Verification items for the finished model (mm, model axes). Give positions to 0.01 mm unless a question says otherwise; leave off trailing zeros. Write each loop counter-clockwise with the first axis right and the second up, starting at its lowest first coordinate (ties: lowest second). Pieces come first, ordered by that corner, then holes. Notation, with made-up numbers: (74, 81.25) - (118, 81.25) arc R20 ccw to (118, 97.25) - close; hole circle Ø6 at (-35.5, -16). An arc over 180 degrees is marked (long way). Put each result on its own line as item: value.
from build123d import *

# Parameters (mm, degrees)
CROQUIS1_W              = 10
CROQUIS1_H              = 40
SALIENTE_EXTRUIR1_DEPTH = 30.26
CROQUIS2_R              = 4
CORTAR_EXTRUIR1_DEPTH   = 30.26
CROQUIS5_R              = 4
CORTAR_EXTRUIR2_DEPTH   = 15.13


with BuildPart() as part:
    # Croquis1 → Saliente-Extruir1 (new body)
    with BuildSketch(Plane(origin=(0, 0, 0), x_dir=(1, 0, 0), z_dir=(0, 1, 0))):
        Rectangle(CROQUIS1_W, CROQUIS1_H)
    extrude(amount=SALIENTE_EXTRUIR1_DEPTH)

    # Croquis2 → Cortar-Extruir1 (cut)
    with BuildSketch(Plane(origin=(0, 0, 0), x_dir=(1, 0, 0), z_dir=(0, 1, 0))):
        with Locations(Location((0, -10, 0), (0, 0, 90))):
            Circle(CROQUIS2_R)
        with Locations(Location((0, 10, 0), (0, 0, 90))):
            Circle(CROQUIS2_R)
    extrude(amount=CORTAR_EXTRUIR1_DEPTH, mode=Mode.SUBTRACT)

    # Croquis5 → Cortar-Extruir2 (cut, symmetric)
    with BuildSketch(Plane(origin=(0, 0, 0), x_dir=(0, 0, -1), z_dir=(1, 0, 0))):
        with Locations((0, 15.13)):
            Circle(CROQUIS5_R)
    extrude(amount=CORTAR_EXTRUIR2_DEPTH, both=True, mode=Mode.SUBTRACT)


solid = part.part
Q1. Go/stop test with a flat-tipped pin: pin 1 Ø7 at (y, z) = (15.13, 0) entering from -X. Record where the tip stops, or that it passes through.
Answers follow:
pin 1: passes through
Q2. Section check C-C, the plane z = 0. Record the cut outline in (x, y), plus the area to 3 significant figures.
Answers follow:
outline: (-5, 0) - (5, 0) - (5, 11.13) - (-5, 11.13) - close; (-5, 19.13) - (5, 19.13) - (5, 30.26) - (-5, 30.26) - close
area: 223 mm2
Q3. Release check for a two-part mould opening along Z. For faces 1 (the face through (0.1, 19.1, 0.5)), 2 (the face through (0, 0, 0)), 3 (the face through (0, 15, 20)) record: released by +Z, released by -Z, zero draft, split by the parting line, or undercut.
Answers follow:
face 1: undercut
face 2: zero draft
face 3: released by +Z
Q4. Scan lines: line 1 along Z through (x, y) = (-0.25, 24); line 2 along X through (y, z) = (9.5, -10); line 3 along Z through (x, y) = (1, 29). Record each from-to range of solid material in increasing order.
Answers follow:
line 1: z = -20 to -13.99, -6.01 to 6.01, 13.99 to 20
line 2: x = -5 to -4, 4 to 5
line 3: z = -20 to -13.87, -6.13 to 6.13, 13.87 to 20
Q5. Section check D-D, the plane y = 9. Record the cut outline in (x, z).
Answers follow:
outline: (-5, -20) - (5, -20) - (5, 20) - (-5, 20) - close; hole circle Ø8 at (0, -10); hole circle Ø8 at (0, 10)
Q6. Section check A-A, the plane x = 0. Record the cut outline in (y, z), plus the area to 3 significant figures.
Answers follow:
outline: (0, -20) - (30.26, -20) - (30.26, -14) - (0, -14) - close; (0, -6) - (30.26, -6) - (30.26, 6) - (0, 6) - close; (0, 14) - (30.26, 14) - (30.26, 20) - (0, 20) - close; hole circle Ø8 at (15.13, 0)
area: 676 mm2
Q7. Section check B-B, the plane y = 15.13. Record the cut outline in (x, z), plus the area to 3 significant figures.
Answers follow:
outline: (-5, -20) - (5, -20) - (5, -4) - (-5, -4) - close; (-5, 4) - (5, 4) - (5, 20) - (-5, 20) - close; hole circle Ø8 at (0, -10); hole circle Ø8 at (0, 10)
area: 219 mm2
